Source: CAD feature listing. Evaluate the final solid. Frame: model axes, mm. Face numbers are marked on the shaded views. Round coordinates to 2 decimals unless told otherwise and drop trailing zeros. Order: outer loops, then holes, each group sorted by start corner. A loop starts at its lowest first (then second) coordinate and runs counter-clockwise, first axis right, second up. Notation, with made-up numbers: (89.5, 5) -> (108.5, 5) arc R20 ccw to (108.5, 37) -> close; hole circle Ø9 at (0, 70.5). An arc over 180 degrees is marked (long way). Answer as CSV lines item,"result".
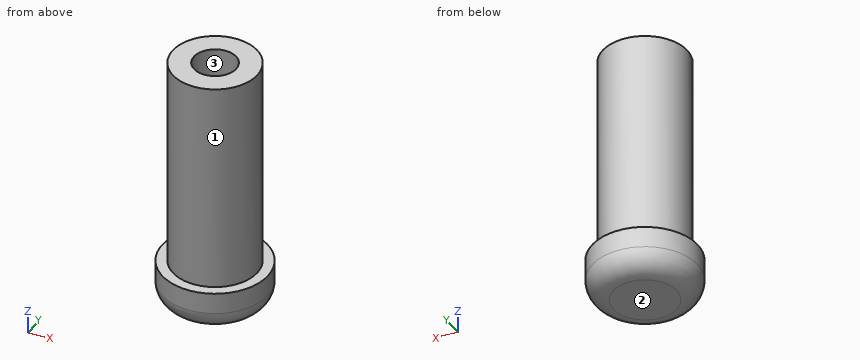
from build123d import *

# Parameters (mm, degrees)
ESQUISSE1_R        = 2.5
BOSS_EXTRU_1_DEPTH = 2
ESQUISSE2_R        = 2
ESQUISSE2_R_2      = 1
BOSS_EXTRU_2_DEPTH = 10
CONG_1_R           = 1


with BuildPart() as part:
    # Esquisse1 → Boss.-Extru.1 (new body)
    with BuildSketch(Plane.XY):
        Circle(ESQUISSE1_R)
    extrude(amount=BOSS_EXTRU_1_DEPTH)

    # Esquisse2 → Boss.-Extru.2 (add)
    with BuildSketch(Plane.XY.offset(2)):
        Circle(ESQUISSE2_R)
        Circle(ESQUISSE2_R_2, mode=Mode.SUBTRACT)
    extrude(amount=BOSS_EXTRU_2_DEPTH)

    # Congé1
    cong_1_edges = [part.edges().sort_by_distance(p)[0] for p in [
        (-2.5, 0, 0),
    ]]
    fillet(cong_1_edges, radius=CONG_1_R)


solid = part.part
1. Section query D-D on z = 1.5. Return loops of the section in (x, y).
Results below:
outline,"circle Ø5 at (0, 0)"
2. Mould query, pull axis Y, two halves, no side actions, for the marked faces 1, 2 and 3. Classes: released by +Y, released by -Y, zero draft, split by the parting line, or undercut.
Results below:
face 1,"split by the parting line"
face 2,"zero draft"
face 3,"undercut"
3. Line query: L1, parallel to Y at x = 0, z = 9.25; L2, parallel to Z at x = -0.85, y = -1.3; L3, parallel to Y at x = 0.6, z = 6.25. Output: solid intervals per line, ascending. Write a range as [from, to].
Results below:
L1,"[-2, -1], [1, 2]"
L2,"[0, 12]"
L3,"[-1.91, -0.8], [0.8, 1.91]"
4. Pin query (flat end, axial travel): pin 1 (0.6 mm diameter, centred on x = 0, y = 0.5, fed in from +Z); pin 2 (2 mm diameter, centred on x = 1, z = 4, fed in from -Y). Return the tip coordinate at first contact, or that it passes through.
Results below:
pin 1,"z = 2"
pin 2,"y = -2"
5. Section query A-A on z = 7.5. Return loops of the section in (x, y), and give its area (3 significant figures).
Results below:
outline,"circle Ø4 at (0, 0); hole circle Ø2 at (0, 0)"
area,"9.42 mm2"
6. Section query B-B on x = 0. Return loops of the section in (y, z).
Results below:
outline,"(-2.5, 1) arc R1 ccw to (-1.5, 0) -> (1.5, 0) arc R1 ccw to (2.5, 1) -> (2.5, 2) -> (2, 2) -> (2, 12) -> (1, 12) -> (1, 2) -> (-1, 2) -> (-1, 12) -> (-2, 12) -> (-2, 2) -> (-2.5, 2) -> close"
